Design review of the part built by this model. Coordinates are the model's own, in mm. Coordinates: 2 decimals unless noted, no trailing zeros. Answer in a Markdown table with one row per item. Add a question column.
(1) We need section A-A, the plane y = 49. Give the number of separate pieces and of enclosed holes in the cut face, plus the area to 3 significant figures.
(2) Clearance check with flat-ended pins moving along their axes: pin 1 (1.5 mm diameter, centred on y = -1.5, z = 1, fed in from +X); pin 2 (1 mm diameter, centred on y = 17.5, z = 1.5, fed in from +X); pin 3 (1.5 mm diameter, centred on x = 85.5, z = 1, fed in from -Y); pin 4 (1 mm diameter, centred on x = 47, y = 54, fed in from -Z). State where each tip first meets the part, or that it passes through.
(3) To check wall thickness, follow L1, parallel to X at y = 54, z = 2.15; L2, parallel to X at y = 55, z = 2.65; L3, parallel to Y at x = 57.5, z = 0.85. State the ranges of each line that lie inside material, in increasing order. Write a range as [from, to].
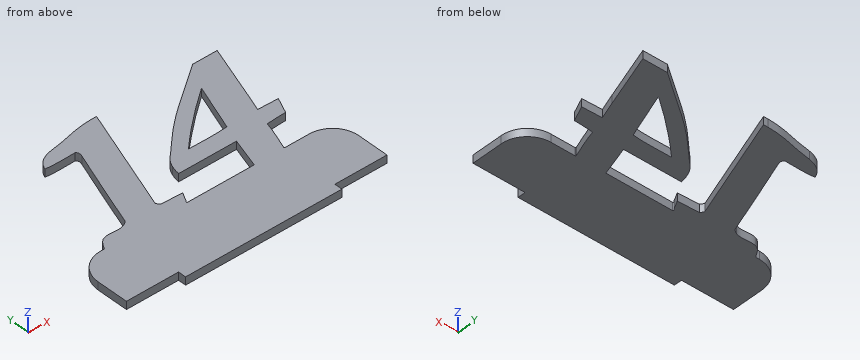
from build123d import *

# Parameters (mm, degrees)
BOSS_EXTRUDE1_DEPTH = 3
FILLET1_R           = 10
FILLET2_R           = 0.2


with BuildPart() as part:
    # Sketch1 → Boss-Extrude1 (new body)
    with BuildSketch(Plane.XY):
        with BuildLine():
            Line((42.749612228, 22.000000982), (68.900263663, 22.000000982))
            Line((68.900263663, 22.000000982), (72.438655427, 33.449873816))
            Line((72.438655427, 33.449873816), (50.272900931, 33.449873816))
            add(Edge.make_bspline(
                [(50.272900931, 33.449873816), (50.399701069, 35.232060422), (51.07430828, 36.890061462)],
                knots=[0, 0, 0, 1, 1, 1], degree=2))
            add(Edge.make_bspline(
                [(51.07430828, 36.890061462), (51.325314504, 37.69426052), (51.918420301, 38.823627057), (52.965393254, 40.197356727), (55.040325227, 42.226401797), (56.906069545, 43.842187727), (58.267427905, 45.334158413)],
                knots=[0, 0, 0, 0, 0.224443411, 0.338858347, 0.460950835, 1, 1, 1, 1], degree=3))
            add(Edge.make_bspline(
                [(58.267427905, 45.334158413), (60.384790067, 47.521422491), (63.79764632, 50.686490857), (68.693222774, 54.688016487), (72.643154035, 57.622122808), (76.561208747, 60.443533866), (81.264828304, 63.875801937), (84.634451747, 66.35024823), (86.766255114, 67.949482885)],
                knots=[0, 0, 0, 0, 0.250612348, 0.382931529, 0.520503025, 0.655730691, 0.780544062, 1, 1, 1, 1], degree=3))
            Line((86.766255114, 67.949482885), (96.1876781, 67.949482885))
            Line((96.1876781, 67.949482885), (89.014104997, 46.917426591))
            Line((89.014104997, 46.917426591), (86.629429469, 40.173876943))
            Line((86.629429469, 40.173876943), (94.350305153, 39.919772174))
            Line((94.350305153, 39.919772174), (91.652885294, 33.84080423))
            add(Edge.make_bspline(
                [(91.652885294, 33.84080423), (90.615751555, 33.849650126), (88.151293743, 33.72895626), (85.689091845, 33.579119519), (84.264300462, 33.449873816)],
                knots=[0, 0, 0, 0, 0.420206299, 1, 1, 1, 1], degree=3))
            add(Edge.make_bspline(
                [(84.264300462, 33.449873816), (83.751919692, 31.362918248), (82.707539096, 28.321707646), (81.319432158, 24.539092544), (80.676394779, 22.768772837), (80.402865584, 22.000000982)],
                knots=[0, 0, 0, 0, 0.502209297, 0.752080888, 0.943038063, 0.943038063, 0.943038063, 0.943038063], degree=3))
            Line((80.402865584, 22.000000982), (90.110220598, 22.000000982))
            Line((90.110220598, 22.000000982), (100, 22.000000982))
            Line((100, 22.000000982), (100, 0))
            Line((100, 0), (80, 0))
            Line((80, 0), (80, -3))
            Line((80, -3), (20, -3))
            Line((20, -3), (20, 0))
            Line((20, 0), (0, 0))
            Line((0, 0), (0, 22.000000982))
            Line((0, 22.000000982), (11.406772984, 22.000000982))
            add(Edge.make_bspline(
                [(11.406772984, 22.000000982), (11.481923411, 22.128324781), (11.803942066, 22.690265443), (12.606466874, 24.1299098), (13.601086209, 25.299520611), (14.541861056, 25.728998132)],
                knots=[0.174411648, 0.174411648, 0.174411648, 0.174411648, 0.24891213, 0.498932816, 1, 1, 1, 1], degree=3))
            add(Edge.make_bspline(
                [(14.541861056, 25.728998132), (15.88322935, 26.248262142), (18.633967114, 25.973494082), (21.403300538, 25.817845983), (22.712306717, 26.393579836)],
                knots=[0, 0, 0, 0, 0.501451854, 1, 1, 1, 1], degree=3))
            add(Edge.make_bspline(
                [(22.712306717, 26.393579836), (23.593849654, 26.784092389), (24.295574895, 27.449091955)],
                knots=[0, 0, 0, 1, 1, 1], degree=2))
            add(Edge.make_bspline(
                [(24.295574895, 27.449091955), (26.077870774, 32.484264955), (29.602867976, 42.60706621), (33.291895969, 52.671262962), (35.124347373, 57.726652549)],
                knots=[0, 0, 0, 0, 0.498322561, 1, 1, 1, 1], degree=3))
            add(Edge.make_bspline(
                [(35.124347373, 57.726652549), (35.307524439, 58.224190762), (35.602710566, 59.190766536), (35.150116794, 60.102162008), (34.792056521, 60.306793284)],
                knots=[0, 0, 0, 0, 0.581397084, 1, 1, 1, 1], degree=3))
            add(Edge.make_bspline(
                [(34.792056521, 60.306793284), (32.875335639, 60.340590356), (29.070344759, 60.156681953), (25.25736304, 60.26141883), (23.376888421, 60.502258491)],
                knots=[0, 0, 0, 0, 0.503014916, 1, 1, 1, 1], degree=3))
            add(Edge.make_bspline(
                [(23.376888421, 60.502258491), (23.608850931, 61.169430986), (24.093094541, 62.118385021), (25.011088656, 63.179121193), (25.784372398, 63.90164623), (26.73233409, 64.45535482), (28.159352101, 65.138054442), (29.35140978, 65.452871316), (30.179077631, 65.584353878)],
                knots=[0, 0, 0, 0, 0.237267367, 0.352023708, 0.469658656, 0.590380818, 0.718477308, 1, 1, 1, 1], degree=3))
            add(Edge.make_bspline(
                [(30.179077631, 65.584353878), (33.291343657, 65.982791022), (37.153111251, 66.834794979), (41.774910805, 67.914609184), (44.8548119, 68.397084929), (47.147903193, 68.544635368), (48.650539711, 68.555425028)],
                knots=[0, 0, 0, 0, 0.501477793, 0.632810111, 0.759518477, 1, 1, 1, 1], degree=3))
            add(Edge.make_bspline(
                [(48.650539711, 68.555425028), (48.859035932, 68.555425028), (49.451947061, 68.555425028), (50.044858189, 68.555425028), (50.429273097, 68.555425028)],
                knots=[0, 0, 0, 0, 0.351648352, 1, 1, 1, 1], degree=3))
            Line((50.429273097, 68.555425028), (36.179859492, 27.918208452))
            add(Edge.make_bspline(
                [(36.179859492, 27.918208452), (36.126676837, 27.718411957), (36.458316573, 27.208718898), (36.736006921, 26.725936024), (37.039906404, 26.452219398)],
                knots=[0, 0, 0, 0, 0.324502414, 1, 1, 1, 1], degree=3))
            Line((37.039906404, 26.452219398), (45.210352065, 26.139475067))
            add(Edge.make_bspline(
                [(45.210352065, 26.139475067), (44.6154125, 25.12625594), (44.070252391, 23.804016563), (43.219476455, 22.414888166), (42.889953696, 22.11142887), (42.749612228, 22.000000982)],
                knots=[0, 0, 0, 0, 0.504343167, 0.619768133, 0.696711259, 0.696711259, 0.696711259, 0.696711259], degree=3))
        make_face()
        with BuildLine():
            add(Edge.make_bspline(
                [(81.293229312, 58.117582963), (77.336378308, 55.190834109), (69.966290168, 49.375200463), (63.02434641, 43.054636478), (59.850696083, 39.919772174)],
                knots=[0, 0, 0, 0, 0.524587428, 1, 1, 1, 1], degree=3))
            add(Edge.make_bspline(
                [(59.850696083, 39.919772174), (62.347046703, 39.956138517), (67.338663055, 39.755607803), (72.337038175, 39.898913575), (74.823330954, 40.173876943)],
                knots=[0, 0, 0, 0, 0.499665743, 1, 1, 1, 1], degree=3))
            add(Edge.make_bspline(
                [(74.823330954, 40.173876943), (75.929225459, 43.166496772), (78.017470904, 49.172207513), (80.19988778, 55.144320848), (81.293229312, 58.117582963)],
                knots=[0, 0, 0, 0, 0.501754487, 1, 1, 1, 1], degree=3))
        make_face(mode=Mode.SUBTRACT)
    extrude(amount=BOSS_EXTRUDE1_DEPTH)

    # Fillet1
    fillet1_edges = [part.edges().sort_by_distance(p)[0] for p in [
        (100, 22.000000982, 1.5),
        (0, 22.000000982, 1.5),
    ]]
    fillet(fillet1_edges, radius=FILLET1_R)

    # Fillet2
    fillet2_edges = [part.edges().sort_by_distance(p)[0] for p in [
        (80.402865584, 22.000000982, 1.5),
        (42.749612228, 22.000000982, 1.5),
        (68.900263663, 22.000000982, 1.5),
        (11.406772984, 22.000000982, 1.5),
    ]]
    fillet(fillet2_edges, radius=FILLET2_R)


solid = part.part
Responses:
| question | item | result |
|---|---|---|
| 1 | separate pieces | 3 |
| 1 | enclosed holes | 0 |
| 1 | area | 93.3 mm2 |
| 2 | pin 1 | stops at x = 80 |
| 2 | pin 2 | stops at x = 98.66 |
| 2 | pin 3 | stops at y = 0 |
| 2 | pin 4 | passes through |
| 3 | L1 | x = [33.77, 45.33], [67.88, 75.89], [79.79, 91.43] |
| 3 | L2 | x = [34.13, 45.68], [69.16, 77.18], [80.15, 91.77] |
| 3 | L3 | y = [-3, 22], [33.45, 44.53] |
